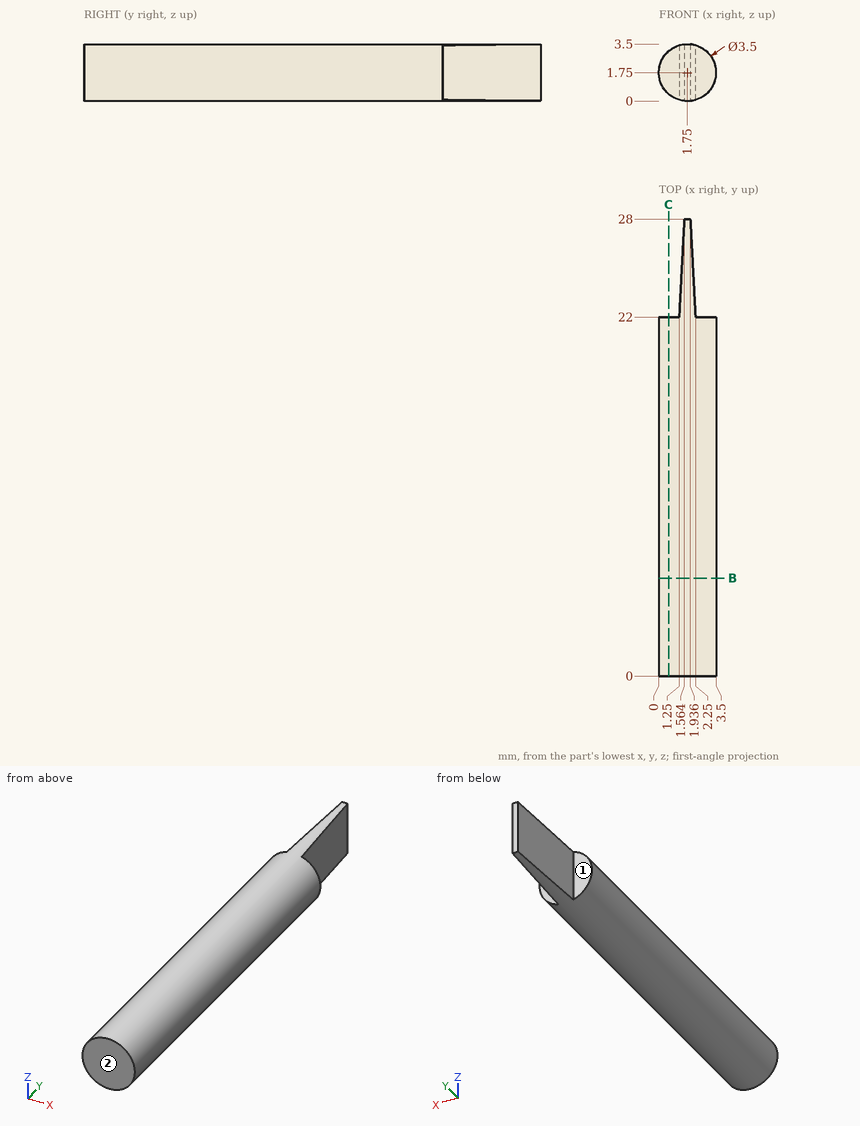
Study the drawing (mm; zero at the part's minimum x, y, z) and answer. A direction names the side the tool comes from. Give positions to 0.01 mm unless a question says otherwise; leave off trailing zeros. Write each loop counter-clockwise with the first axis right and the second up, starting at its lowest first coordinate (ties: lowest second). Pieces come first, ordered by that corner, then holes.
Item 1: Which of the six approach directions +Z, -Z, +X, -X, +Y, -Y give full straight-line access (tool end or side, diameter ignored) to the marked faces 1 and 2?
Item 2: Section B-B, the plane y = 6 is taken. Write down the section's boundary in (x, z).
Item 3: Section C-C, the plane x = 0.6 is taken. Write down the section's boundary in (y, z).
Item 4: Find the intervals of material crossed by line 1 along Y through (x, z) = (3.2, 1); line 2 along Z through (x, y) = (2.25, 15.25); line 3 along Z through (x, y) = (0.7, 12), in increasing order.
Item 5: Flat-ended cylindrical pins translate along their axes: P1, Ø1, axis at x = 0.5, z = 2, coming from the +Y side; P2, Ø1, axis at x = 1, y = 7.5, coming from the -Z side. Find the tip coordinate at first contact, or state that the pin passes through.
Completed:
1. face 1: +Z, -Z, -X, +Y
1. face 2: +Z, -Z, +X, -X, -Y
2. outline: circle Ø3.5 at (1.75, 1.75)
3. outline: (0, 0.43) - (22, 0.43) - (22, 3.07) - (0, 3.07) - close
4. line 1: y = 0 to 22
4. line 2: z = 0.07 to 3.43
4. line 3: z = 0.35 to 3.15
5. P1: stops at y = 22
5. P2: stops at z = 0.02
